Check sheet for the drawn part. Datum: minimum x, y, z corner. Units: mm. A direction names the side the tool comes from. Round coordinates to 2 decimals unless told otherwise and drop trailing zeros. Write each loop counter-clockwise with the first axis right and the second up, starting at its lowest first coordinate (ties: lowest second). Pieces come first, ordered by that corner, then holes. Notation, with made-up numbers: (20.5, 32.5) - (52.5, 32.5) arc R19 cw to (52.5, 42.5) - close; hole circle Ø6 at (19.5, 62.5). An arc over 180 degrees is marked (long way). Answer as a JSON object with one key per item and string values.
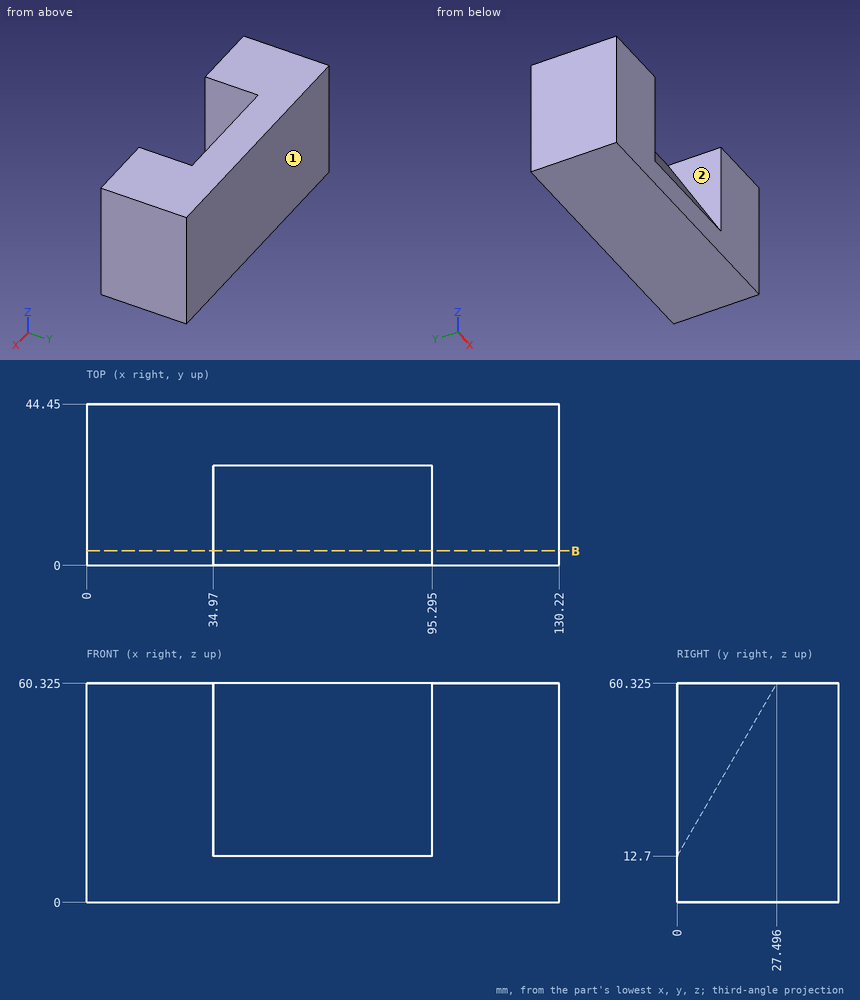
1. Access from +Z, -Z, +X, -X, +Y, -Y to the whole of each face (thin tool, end or side, straight path). Record for the marked faces 1 and 2.
Completed:
{"face 1": "+Z, -Z, +X, -X, +Y", "face 2": "+Z, -Y"}
2. Cross-section at B-B (y = 4). Record the boundary of the cut face in (x, z) (1 decimal).
Completed:
{"outline": "(0, 0) - (130.2, 0) - (130.2, 60.3) - (95.3, 60.3) - (95.3, 19.6) - (35, 19.6) - (35, 60.3) - (0, 60.3) - close"}
3. Go/stop test with a flat-tipped pin: pin 1 (4 mm diameter, centred on x = 78.5, z = 34.5, fed in from -Y). Record where the tip stops, or that it passes through.
Completed:
{"pin 1": "stops at y = 11.43"}
4. Material ranges on probe 1 along X at (y, z) = (2.5, 33) (1 decimal); probe 2 along Z at (x, y) = (94, 6) (1 decimal); probe 3 along Z at (x, y) = (65.5, 9.5) (1 decimal), recorded low to high. Write a range as from..to.
Completed:
{"probe 1": "x = 0..35, 95.3..130.2", "probe 2": "z = 0..23.1", "probe 3": "z = 0..29.2"}
